CAD build for the part. Positions are in the model's coordinates, mm. A direction names the side the tool comes from. Round coordinates to 2 decimals unless told otherwise and drop trailing zeros. Order: outer loops, then holes, each group sorted by start corner. A loop starts at its lowest first (then second) coordinate and runs counter-clockwise, first axis right, second up. Notation, with made-up numbers: (53, -29.5) -> (76, -29.5) arc R19 ccw to (76, -3.5) -> close; hole circle Ø6 at (65.25, 85). An arc over 180 degrees is marked (long way). Return JSON: item names as keys, results as strings. Group by question number.
Q1. Cut at D-D (x = 25.5). Write the cut outline in (y, z), then the cut area to 3 significant figures.
Q2. Cut at B-B (z = 2). Write the cut outline in (x, y), then the cut area to 3 significant figures.
Q3. Cut at A-A (y = 53.5). Write the cut outline in (x, z), then the cut area to 3 significant figures.
Q4. Mould opens along Z. For faces 6 (the flat face through (2.5, 16, 9)), 7 (the flat face through (37, 4, 9)), 8 (the flat face through (2, 39, 17)) say: +Z half, -Z half, draft (parallel to the pull), parting line (faces both ways), or undercut.
Q5. Which spindle directions (+Z, -Z, +X, -X, +Y, -Y) get a long thin tool onto all of the face, cutting with end or side? Do faces 1 (the flat face through (17, 80, 6)), 2 (the cylindrical face through (20.86, 77.46, 16.1)), 3 (the flat face through (20, 50, 10)), 4 (the flat face through (36, 63, 9)), 5 (the flat face through (3.77, 17.86, 11.27)). Say none if no direction does.
Q6. Probe line 1 along X through (y, z) = (52.5, 7.5); line 2 along Y through (x, z) = (22, 16); line 3 along Y through (x, z) = (12, 2.5). List the from-to ranges inside material, lowest first.
Q7. Cut at C-C (x = 13). Write the cut outline in (y, z).
Q8. Flat gauge pins, fed straight in: pin 1 (4 mm diameter, centred on x = 32.5, z = 5, fed in from +Y); pin 2 (8 mm diameter, centred on x = 13, y = 53, fed in from +Z); pin 3 (5 mm diameter, centred on x = 21, z = 7.5, fed in from -Y); pin 4 (10 mm diameter, centred on x = 20.5, y = 43, fed in from +Z). Where does each tip first touch, or does it go through?
from build123d import *

# Parameters (mm, degrees)
SKETCH1_W             = 5
SKETCH1_H             = 17
BOSS_EXTRUDE1_DEPTH   = 80
BOSS_EXTRUDE1_2_DEPTH = 80
CUT_EXTRUDE1_DEPTH    = 2.5
SKETCH7_W             = 17
SKETCH7_H             = 4
CUT_EXTRUDE4_DEPTH    = 5
SKETCH8_R             = 2
CUT_EXTRUDE5_DEPTH    = 5
BOSS_EXTRUDE3_REACH   = 91.359
SKETCH9_W             = 7
SKETCH9_H             = 5
SKETCH10_W            = 10
SKETCH10_H            = 5
BOSS_EXTRUDE4_DEPTH   = 16
FILLET3_R             = 3
BOSS_EXTRUDE5_DEPTH   = 17
FILLET4_R             = 2
FILLET5_R             = 15


with BuildPart() as part:
    # Sketch1 → Boss-Extrude1 (new body)
    with BuildSketch(Plane(origin=(0, 0, 0), x_dir=(1, 0, 0), z_dir=(0, 1, 0))):
        with Locations((2.5, -8.5)):
            Rectangle(SKETCH1_W, SKETCH1_H)
    extrude(amount=BOSS_EXTRUDE1_DEPTH)

    # Sketch2 → Cut-Extrude1 (cut)
    with BuildSketch(Plane(origin=(5, 0, 0), x_dir=(0, 0, -1), z_dir=(1, 0, 0))):
        with BuildLine():
            Line((-10.75, 25.267799715), (-11.807189139, 10.25))
            ThreePointArc((-11.807189139, 10.25), (-8.5, 12), (-5.192810861, 10.25))
            Line((-5.192810861, 10.25), (-6.25, 25.267799715))
            ThreePointArc((-6.25, 25.267799715), (-8.5, 27.517799715), (-10.75, 25.267799715))
        make_face()
        with BuildLine():
            ThreePointArc((-5.192810861, 10.25), (-8.5, 12), (-11.807189139, 10.25))
            Line((-11.807189139, 10.25), (-11.807189139, 5.75))
            ThreePointArc((-11.807189139, 5.75), (-8.5, 4), (-5.192810861, 5.75))
            Line((-5.192810861, 5.75), (-5.192810861, 10.25))
        make_face()
        with BuildLine():
            Line((-11.807189139, 5.75), (-11.807189139, 10.25))
            ThreePointArc((-11.807189139, 10.25), (-12.5, 8), (-11.807189139, 5.75))
        make_face()
        with BuildLine():
            ThreePointArc((-4.5, 8), (-4.677124344, 9.177124344), (-5.192810861, 10.25))
            Line((-5.192810861, 10.25), (-5.192810861, 5.75))
            ThreePointArc((-5.192810861, 5.75), (-4.677124344, 6.822875656), (-4.5, 8))
        make_face()
    extrude(amount=-CUT_EXTRUDE1_DEPTH, mode=Mode.SUBTRACT)


with BuildPart() as body_2:
    # Sketch1 → Boss-Extrude1 2 (new body)
    with BuildSketch(Plane(origin=(0, 0, 0), x_dir=(1, 0, 0), z_dir=(0, 1, 0))):
        with Locations((38.5, -8.5)):
            Rectangle(SKETCH1_W, SKETCH1_H)
    extrude(amount=BOSS_EXTRUDE1_2_DEPTH)

    # Sketch7 → Cut-Extrude4 (cut)
    with BuildSketch(Plane(origin=(41, 0, 0), x_dir=(0, 0, -1), z_dir=(1, 0, 0))):
        with Locations((-8.5, 2)):
            Rectangle(SKETCH7_W, SKETCH7_H)
    extrude(amount=-CUT_EXTRUDE4_DEPTH, mode=Mode.SUBTRACT)

    # Sketch8 → Cut-Extrude5 (cut)
    with BuildSketch(Plane(origin=(41, 0, 0), x_dir=(0, 0, -1), z_dir=(1, 0, 0))):
        with Locations((-8.5, 8)):
            Circle(SKETCH8_R)
    extrude(amount=-CUT_EXTRUDE5_DEPTH, mode=Mode.SUBTRACT)

    # Sketch9 → Boss-Extrude3 (add, up to next)
    with BuildSketch(Plane(origin=(5, 0, 0), x_dir=(0, 0, -1), z_dir=(1, 0, 0)), mode=Mode.PRIVATE) as boss_extrude3_sk1:
        with Locations((-3.5, 77.5)):
            Rectangle(SKETCH9_W, SKETCH9_H)
    boss_extrude3_tool1 = extrude(boss_extrude3_sk1.sketch, amount=BOSS_EXTRUDE3_REACH, mode=Mode.PRIVATE) - body_2.part
    # Sketch9 → Boss-Extrude3 (add, up to next)
    with BuildSketch(Plane(origin=(5, 0, 0), x_dir=(0, 0, -1), z_dir=(1, 0, 0)), mode=Mode.PRIVATE) as boss_extrude3_sk2:
        with Locations((-3.5, 49.5)):
            Rectangle(SKETCH9_W, SKETCH9_H)
    boss_extrude3_tool2 = extrude(boss_extrude3_sk2.sketch, amount=BOSS_EXTRUDE3_REACH, mode=Mode.PRIVATE) - body_2.part

    add(part.part)  # Boss-Extrude3 merges part
    add(boss_extrude3_tool1.solids().sort_by_distance((5, 77.5, 3.5))[0])
    add(boss_extrude3_tool2.solids().sort_by_distance((5, 49.5, 3.5))[0])

    # Sketch10 → Boss-Extrude4 (add)
    with BuildSketch(Plane.ZY.offset(-36)):
        with Locations((12, 77.5)):
            Rectangle(SKETCH10_W, SKETCH10_H)
        with Locations((12, 49.5)):
            Rectangle(SKETCH10_W, SKETCH10_H)
    extrude(amount=BOSS_EXTRUDE4_DEPTH)

    # Fillet3
    # the kernel refuses this fillet: 3 mm, written as the material it takes off along each edge
    with BuildSketch(Plane(origin=(41, 80, -7.5), x_dir=(0, -1, 0), z_dir=(0, 0, 1)), Plane(origin=(41, 4, 24.5), x_dir=(0, 1, 0), z_dir=(0, 0, -1))) as fillet3_piece_1:
        with BuildLine():
            CenterArc((FILLET3_R, -FILLET3_R), FILLET3_R, 90, 90)
            Line((0, -FILLET3_R), (0, 0))
            Line((0, 0), (FILLET3_R, 0))
        make_face()
    extrude(amount=32, mode=Mode.SUBTRACT)
    with BuildSketch(Plane(origin=(0, 80, 24.5), x_dir=(1, 0, 0), z_dir=(0, 0, -1)), Plane(origin=(0, 0, 24.5), x_dir=(0, 1, 0), z_dir=(0, 0, -1))) as fillet3_piece_2:
        with BuildLine():
            CenterArc((FILLET3_R, FILLET3_R), FILLET3_R, 180, 90)
            Line((0, FILLET3_R), (0, 0))
            Line((0, 0), (FILLET3_R, 0))
        make_face()
    extrude(amount=32, mode=Mode.SUBTRACT)
    with BuildSketch(Plane(origin=(20, 67.5, 17), x_dir=(0, 0, -1), z_dir=(0, 1, 0))) as fillet3_piece_3:
        with BuildLine():
            CenterArc((FILLET3_R, -FILLET3_R), FILLET3_R, 90, 90)
            Line((0, -FILLET3_R), (0, 0))
            Line((0, 0), (FILLET3_R, 0))
        make_face()
    extrude(amount=20, mode=Mode.SUBTRACT)
    with BuildSketch(Plane(origin=(20, 39.5, 17), x_dir=(1, 0, 0), z_dir=(0, 1, 0))) as fillet3_piece_4:
        with BuildLine():
            CenterArc((FILLET3_R, FILLET3_R), FILLET3_R, 180, 90)
            Line((0, FILLET3_R), (0, 0))
            Line((0, 0), (FILLET3_R, 0))
        make_face()
    extrude(amount=20, mode=Mode.SUBTRACT)

    # Sketch12 → Boss-Extrude5 (add, through all)
    with BuildSketch(Plane.XY.offset(17)):
        with BuildLine():
            Line((17.07120829, 119.558177775), (35.709852909, 114.232850741))
            ThreePointArc((35.709852909, 114.232850741), (40.614477912, 95.937468732), (41, 77))
            Line((41, 77), (30.5, 80))
            ThreePointArc((30.5, 80), (28.882999649, 101.509498789), (17.07120829, 119.558177775))
        make_face()
    extrude(amount=-BOSS_EXTRUDE5_DEPTH)

    # Fillet4
    fillet4_edges = [body_2.edges().sort_by_distance(p)[0] for p in [
        (17.07120829, 119.558177775, 8.5),
    ]]
    fillet(fillet4_edges, radius=FILLET4_R)

    # Fillet5
    fillet5_edges = [body_2.edges().sort_by_distance(p)[0] for p in [
        (35.709852909, 114.232850741, 8.5),
    ]]
    fillet(fillet5_edges, radius=FILLET5_R)


solid = body_2.part
Solution:
{
 "1": {"outline": "(47, 0) -> (52, 0) -> (52, 17) -> (47, 17) -> close; (75, 0) -> (80, 0) -> (80, 17) -> (75, 17) -> close; (109.03, 0) -> (117.15, 0) -> (117.15, 17) -> (109.03, 17) -> close", "area": "308 mm²"},
 "2": {"outline": "(0, 3) arc R3 ccw to (3, 0) -> (5, 0) -> (5, 47) -> (36, 47) -> (36, 4) -> (38, 4) arc R3 ccw to (41, 7) -> (41, 77) arc R78.6 ccw to (38.51, 105.99) arc R15 ccw to (28.18, 116.38) -> (23.98, 117.58) arc R2 ccw to (21.86, 114.42) arc R43.22 cw to (30.5, 80) -> (3, 80) arc R3 ccw to (0, 77) -> close; hole (5, 52) -> (36, 52) -> (36, 75) -> (5, 75) -> close", "area": "1,480 mm²"},
 "3": {"outline": "(0, 0) -> (5, 0) -> (5, 17) -> (0, 17) -> close; (36, 0) -> (41, 0) -> (41, 17) -> (36, 17) -> close", "area": "170 mm²"},
 "4": {"face 6": "undercut", "face 7": "draft", "face 8": "+Z half"},
 "5": {"face 1": "+Z, -Z, -X", "face 2": "+Z, -Y", "face 3": "+Z, +Y, -Y", "face 4": "+Z, -Z", "face 5": "none"},
 "6": {"line 1": "x = 0 to 5, 36 to 41", "line 2": "y = 47 to 52, 75 to 80, 114.24 to 117.06", "line 3": "y = 47 to 52, 75 to 80"},
 "7": {"outline": "(47, 0) -> (52, 0) -> (52, 7) -> (47, 7) -> close; (75, 0) -> (80, 0) -> (80, 7) -> (75, 7) -> close"},
 "8": {"pin 1": "stops at y = 115.51", "pin 2": "stops at z = 7", "pin 3": "stops at y = 47", "pin 4": "stops at z = 17"}
}
